Build history of the part. All positions in model axes, mm. Face numbers are marked on the shaded views. Round coordinates to 2 decimals unless told otherwise and drop trailing zeros. Write each loop counter-clockwise with the first axis right and the second up, starting at its lowest first coordinate (ties: lowest second). Pieces come first, ordered by that corner, then holes. Notation, with made-up numbers: (7, 44.25) - (26, 44.25) arc R18 ccw to (26, 72.25) - close; hole circle Ø7 at (48.5, 12.5). An arc over 180 degrees is marked (long way). Answer as a JSON object with one key per item and string values. Group by question number.
Item 1: Slice it at C-C, the plane y = -36. List the corners of the cut face in (x, z), then the cut area to 3 significant figures.
Item 2: Flat gauge pins, fed straight in: pin 1 (2.5 mm diameter, centred on y = 56.45, z = 0, fed in from +X); pin 2 (1 mm diameter, centred on y = -5, z = -2.5, fed in from -X). Where does each tip first touch, or does it go through?
Item 3: Two-plate mould, pull along Z, no slides. Class the marked faces 1 and 2: +Z half, -Z half, draft (parallel to the pull), parting line (faces both ways), or undercut.
Item 4: Slice it at B-B, the plane x = 2.25. List the corners of the cut face in (y, z).
Item 5: Slice it at A-A, the plane z = 0. List the corners of the cut face in (x, y), then the cut area to 3 significant figures.
Item 6: Probe line 1 (Y direction, x = 3.5, z = -0.25); line 2 (Y direction, x = 0.5, z = 0.75); line 3 (X direction, y = -43.5, z = 0.25). List the from-to ranges inside material, lowest first. Write a range as from..to.
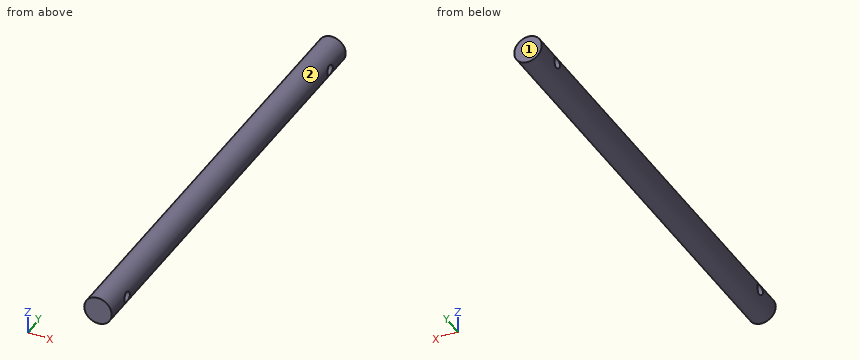
from build123d import *

# Parameters (mm, degrees)
SKETCH1_R           = 3.937
BOSS_EXTRUDE1_DEPTH = 65.0875
SKETCH2_W           = 14.723977987
SKETCH2_H           = 1.524
SKETCH3_W           = 14.493300334
SKETCH3_H           = 1.524


with BuildPart() as part:
    # Sketch1 → Boss-Extrude1 (new, symmetric)
    with BuildSketch(Plane(origin=(0, 0, 0), x_dir=(1, 0, 0), z_dir=(0, 1, 0))):
        with Locations(Location((0, 0, 0), (0, 0, 270))):
            Circle(SKETCH1_R)
    extrude(amount=BOSS_EXTRUDE1_DEPTH, both=True)

    # Sketch2 → Cut-Revolve1 (revolve, cut)
    with BuildSketch(Plane.XY, mode=Mode.PRIVATE) as cut_revolve1_sk:
        with Locations((0.698328764, 57.2135)):
            Rectangle(SKETCH2_W, SKETCH2_H)
    revolve(cut_revolve1_sk.sketch.rotate(Axis((-6.663660229, 56.4515, 0), (1, 0, 0)), 90), axis=Axis((-6.663660229, 56.4515, 0), (1, 0, 0)), mode=Mode.SUBTRACT)

    # Sketch3 → Cut-Revolve2 (revolve, cut)
    with BuildSketch(Plane.XY, mode=Mode.PRIVATE) as cut_revolve2_sk:
        with Locations((0.075239778, -57.2135)):
            Rectangle(SKETCH3_W, SKETCH3_H)
    revolve(cut_revolve2_sk.sketch.rotate(Axis((-7.171410389, -56.4515, 0), (1, 0, 0)), 270), axis=Axis((-7.171410389, -56.4515, 0), (1, 0, 0)), mode=Mode.SUBTRACT)


solid = part.part
Geometry says:
{
 "1": {"outline": "circle Ø7.87 at (0, 0)", "area": "48.7 mm^2"},
 "2": {"pin 1": "passes through", "pin 2": "stops at x = -3.39"},
 "3": {"face 1": "draft", "face 2": "parting line"},
 "4": {"outline": "(-65.09, -3.23) - (65.09, -3.23) - (65.09, 3.23) - (-65.09, 3.23) - close; hole circle Ø3.05 at (-56.45, 0); hole circle Ø3.05 at (56.45, 0)"},
 "5": {"outline": "(-3.94, -65.09) - (3.94, -65.09) - (3.94, -57.98) - (-3.94, -57.98) - close; (-3.94, -54.93) - (3.94, -54.93) - (3.94, 54.93) - (-3.94, 54.93) - close; (-3.94, 57.98) - (3.94, 57.98) - (3.94, 65.09) - (-3.94, 65.09) - close", "area": "977 mm^2"},
 "6": {"line 1": "y = -65.09..-57.95, -54.95..54.95, 57.95..65.09", "line 2": "y = -65.09..-57.78, -55.12..55.12, 57.78..65.09", "line 3": "x = -3.93..3.93"}
}
